Autodesk Inventor part; units mm, degrees
ref_plane "YZ Plane" through (0, 0, 0) normal (1, 0, 0) x (0, 1, 0)
ref_plane "XZ Plane" through (0, 0, 0) normal (0, 1, 0) x (-1, 0, 0)
ref_plane "XY Plane" through (0, 0, 0) normal (0, 0, 1) x (1, 0, 0)
sketch "スケッチ1" plane through (0, 0, 0) normal (1, 0, 0) x (0, 1, 0)
  arc A0 (38.1972, 0) -> (-32.0976, -20.7068) centre (0, 0) ccw
  arc A1 (-37.8876, -435.1467) -> (38.1972, -440) centre (0, -440) ccw
  arc A2 (6.9469, -85.1461) -> (5.5796, -79.1102) centre (-2, -84) ccw
  line L0 (5.5796, -79.1102) -> (-32.0976, -20.7068)
  line L1 (38.1972, -440) -> (38.1972, 0)
  line L2 (6.9469, -85.1461) -> (-37.8876, -435.1467)
  arc A3 (39.2172, 0) -> (-32.9547, -21.2597) centre (0, 0) ccw
  line L3 (-32.9547, -21.2597) -> (4.7225, -79.6632)
  arc A4 (5.9352, -85.0165) -> (4.7225, -79.6632) centre (-2, -84) ccw
  line L4 (5.9352, -85.0165) -> (-38.8993, -435.0171)
  arc A5 (-38.8993, -435.0171) -> (39.2172, -440) centre (0, -440) ccw
  line L5 (39.2172, -440) -> (39.2172, 0)
  arc A6 (37.7172, 0) -> (-31.6942, -20.4466) centre (0, 0) ccw
  line L6 (-31.6942, -20.4466) -> (5.983, -78.85)
  arc A7 (7.423, -85.2071) -> (5.983, -78.85) centre (-2, -84) ccw
  line L7 (7.423, -85.2071) -> (-37.4115, -435.2077)
  arc A8 (-37.4115, -435.2077) -> (37.7172, -440) centre (0, -440) ccw
  line L8 (37.7172, -440) -> (37.7172, 0)
  dimension "d0" = 76.3944
  dimension "d1" = 76.3944
  dimension "d2" = 440
  dimension "d25" = 8
  dimension "d26" = 84
  dimension "d30" = 2
  dimension "d31" = 1.5
  dimension "d32" = 0.48
extrude "押し出し1" add sketch "スケッチ1" along normal mid plane 10 contours L1 A1 L2 A2 L0 A0 | L5 A5 L4 A4 L3 A3
equation "\"d0\" = d1"
properties part number "belt_1" material "ゴム"
For this review, take the finished solid that the model builds, in its own axes (mm). A direction names the side the tool comes from. Give positions to 0.01 mm unless a question says otherwise; leave off trailing zeros. Order: outer loops, then holes, each group sorted by start corner. A loop starts at its lowest first (then second) coordinate and runs counter-clockwise, first axis right, second up. Notation, with made-up numbers: M -16,-31.75 L 3,-31.75 A26 ccw 3,5.25 Z; hole C 51.5,32.25 d8. An arc over 180 degrees is marked long. Answer in a Markdown table with one row per item. Add a question column.
(1) For faces 1 (the face through (0.07, -13.12, -49.24)), 2 (the face through (0.07, -16.17, -257.57)), 3 (the face through (5, -15, -257)), list the 3-axis set-ups (+Z, -Z, +X, -X, +Y, -Y) from which the entire face can be reached by the end or side of a thin tool; tool diameter is ignored.
(2) Consider section D-D on y = 16. State the section outline as (x, z) points, and give its area (3 significant figures).
(3) Consider section B-B on z = -12. State the section outline as (x, y) points, and give its area (3 significant figures).
(4) Consider section A-A on y = -18.5. State the section outline as (x, z) points, and give its area (3 significant figures).
(5) Wall thickness on probe 1 along Z at (x, y) = (2.25, 27.5); probe 2 along Y at (x, z) = (-2, -38); probe 3 along Y at (x, z) = (-1.75, -358.5): over which ranges is each line inside the solid? List them lowest first. Write a range as [from, to].
(6) For pin 1 (1.5 mm diameter, centred on x = -4, y = 17, fed in from +Z); pin 2 (6 mm diameter, centred on x = -2.5, y = 30, fed in from +Z); pin 3 (4 mm diameter, centred on y = -22, z = -279.5, fed in from -X), all flat-tipped, find the tip position at first contact; note any pin that passes through.
(7) Consider section C-C on x = 0. State the section outline as (y, z) points, and give its area (3 significant figures).
(8) Mouldability with a two-part tool opening along Y and no side actions: class faces 4 (the face through (0.07, -10.1, 37.894)), 5 (the face through (-5, -15, -257)), 6 (the face through (0.07, -3.262, -477.576)) as +Y half, -Y half, draft (parallel to the pull), parting line (faces both ways), or undercut.
Evaluation:
| question | item | result |
|---|---|---|
| 1 | face 1 | +X, -X |
| 1 | face 2 | +X, -X, -Y |
| 1 | face 3 | +Z, -Z, +X, +Y, -Y |
| 2 | outline | M -5,-475.8 L 5,-475.8 L 5,-474.16 L -5,-474.16 Z; M -5,34.16 L 5,34.16 L 5,35.8 L -5,35.8 Z |
| 2 | area | 33.0 mm^2 |
| 3 | outline | M -5,-37.34 L 5,-37.34 L 5,-35.76 L -5,-35.76 Z; M -5,37.72 L 5,37.72 L 5,39.22 L -5,39.22 Z |
| 3 | area | 30.8 mm^2 |
| 4 | outline | M -5,-474.58 L 5,-474.58 L 5,-472.87 L -5,-472.87 Z; M -5,-287.58 L 5,-287.58 L 5,-275.77 L -5,-275.77 Z; M -5,-43.67 L 5,-43.67 L 5,-40.9 L -5,-40.9 Z; M -5,32.87 L 5,32.87 L 5,34.58 L -5,34.58 Z |
| 4 | area | 180 mm^2 |
| 5 | probe 1 | z = [-467.96, -465.81], [25.81, 27.96] |
| 5 | probe 2 | y = [-22.16, -20.37], [37.72, 39.22] |
| 5 | probe 3 | y = [-29.1, -27.59], [37.72, 39.22] |
| 6 | pin 1 | stops at z = 35.69 |
| 6 | pin 2 | stops at z = 28.44 |
| 6 | pin 3 | passes through |
| 7 | outline | M -38.9,-435.02 A39.22 ccw long 39.22,-440 L 39.22,0 A39.22 ccw long -32.95,-21.26 L 4.72,-79.66 A8 cw 5.94,-85.02 Z; hole M -37.41,-435.21 A37.72 ccw long 37.72,-440 L 37.72,0 A37.72 ccw long -31.69,-20.45 L 5.98,-78.85 A9.5 cw 7.42,-85.21 Z |
| 7 | area | 1,710 mm^2 |
| 8 | face 4 | parting line |
| 8 | face 5 | draft |
| 8 | face 6 | undercut |
